Autodesk Inventor part; units mm, degrees
ref_plane "YZ Plane" through (0, 0, 0) normal (1, 0, 0) x (0, 1, 0)
ref_plane "XZ Plane" through (0, 0, 0) normal (0, 1, 0) x (-1, 0, 0)
ref_plane "XY Plane" through (0, 0, 0) normal (0, 0, 1) x (1, 0, 0)
sketch "Sketch1" plane through (0, 0, 0) normal (0, 1, 0) x (-1, 0, 0)
  line L0 (3.5, 3.5) -> (-2.5, 3.5)
  line L1 (-2.5, 3.5) -> (-2.5, -3.5)
  line L2 (-2.5, -3.5) -> (3.5, -3.5)
  line L3 (4.5, -3.5) -> (4.5, 3.5)
  line L4 (4.5, 3.5) -> (4.5, 6.5)
  line L5 (4.5, 6.5) -> (1.5, 6.5)
  line L6 (1.5, 6.5) -> (1.5, 5.5)
  line L7 (1.5, 5.5) -> (3.5, 5.5)
  line L8 (3.5, 5.5) -> (3.5, 3.5)
  line L9 (4.5, -3.5) -> (4.5, -6.5)
  line L10 (4.5, -6.5) -> (1.5, -6.5)
  line L11 (1.5, -6.5) -> (1.5, -5.5)
  line L12 (1.5, -5.5) -> (3.5, -5.5)
  line L13 (3.5, -5.5) -> (3.5, -3.5)
  point P0 (0, 0)
  dimension "d2" = 3.5
  dimension "d3" = 4.5
  dimension "d4" = 1
  dimension "d5" = 1
  dimension "d6" = 2
  dimension "d7" = 2
  dimension "d8" = 7
  dimension "d9" = 7
  dimension "d10" = 1
  dimension "d11" = 1
  dimension "d12" = 3
  dimension "d13" = 3
extrude "Extrusion1" add sketch "Sketch1" along normal blind 120
sketch "Sketch2" plane through (-4.5, 0, -6.5) normal (-1, 0, 0) x (0, 0, 1)
  line L0 (0, 0) -> (13, 0)
  line L1 (0, 0) -> (0, 120)
  point P0 (6.5, 0)
  point P1 (6.5, 60)
  dimension "d16" = 60
  dimension "d17" = 6.5
hole "Hole1" at (-4.5, 60, 0) direction (1, 0, 0) diameter 3.5 end through all
properties part number "Stringer cap"
Input: part model. Units: mm. Frame: model coordinates. A direction names the side the tool comes from. Round coordinates to 2 decimals unless told otherwise and drop trailing zeros. Write each loop counter-clockwise with the first axis right and the second up, starting at its lowest first coordinate (ties: lowest second). Pieces come first, ordered by that corner, then holes.
1) Draft query along Z for faces 1 (the flat face through (-3, 59, 6.5)), 2 (the flat face through (-3, 59, -6.5)), 3 (the flat face through (-2, 0, 0)), 4 (the flat face through (0, 59, -3.5)). Return one class per face: pulls with the +Z half, pulls with the -Z half, needs draft (parallel to the pull), parting line crosses it, or undercut.
2) Contact query for flat-ended pins moving along their axis: P1, Ø0.8, axis at y = 58.5, z = 6, coming from the +X side; P2, Ø1.6, axis at y = 78.5, z = 4.5, coming from the +X side; P3, Ø1, axis at x = 0, y = 60, coming from the +Z side. Output: stop coordinate, or through.
3) Reachability of faces 5 (the flat face through (-2, 120, 0)), 6 (the flat face through (-2, 59, 5.5)) from +Z, -Z, +X, -X, +Y, -Y: full face, straight path, thin tool, end or side. Return the list, or none.
4) Ray query, L1, parallel to Z at x = -2.25, y = 41; L2, parallel to Y at x = -1.25, z = 0; L3, parallel to X at y = 70, z = 5.25. Return the intervals inside material, ascending.
5) Cut plane B-B (z = 0). Return the cut outline in (x, y), then the cut area to 4 significant figures.
6) Cut plane D-D (y = 90). Return the cut outline in (x, z).
7) Cut plane C-C (x = -0.5). Return the cut outline in (y, z), then the cut area to 3 significant figures.
8) Cut plane A-A (y = 60). Return the cut outline in (x, z), then the cut area to 3 significant figures.
Geometry says:
1. face 1: pulls with the +Z half
1. face 2: pulls with the -Z half
1. face 3: needs draft
1. face 4: undercut
2. P1: stops at x = -1.5
2. P2: stops at x = -3.5
2. P3: stops at z = 3.5
3. face 5: +Z, -Z, +X, -X, +Y
3. face 6: +X, +Y, -Y
4. L1: z = -6.5 to -5.5, -3.5 to 3.5, 5.5 to 6.5
4. L2: y = 0 to 58.25, 61.75 to 120
4. L3: x = -4.5 to -3.5
5. outline: (-4.5, 0) - (2.5, 0) - (2.5, 58.25) - (-4.5, 58.25) - close; (-4.5, 61.75) - (2.5, 61.75) - (2.5, 120) - (-4.5, 120) - close
5. area: 815.5 mm2
6. outline: (-4.5, -6.5) - (-1.5, -6.5) - (-1.5, -5.5) - (-3.5, -5.5) - (-3.5, -3.5) - (2.5, -3.5) - (2.5, 3.5) - (-3.5, 3.5) - (-3.5, 5.5) - (-1.5, 5.5) - (-1.5, 6.5) - (-4.5, 6.5) - close
7. outline: (0, -3.5) - (120, -3.5) - (120, 3.5) - (0, 3.5) - close; hole circle Ø3.5 at (60, 0)
7. area: 830 mm2
8. outline: (-4.5, -6.5) - (-1.5, -6.5) - (-1.5, -5.5) - (-3.5, -5.5) - (-3.5, -3.5) - (2.5, -3.5) - (2.5, -1.75) - (-4.5, -1.75) - close; (-4.5, 1.75) - (2.5, 1.75) - (2.5, 3.5) - (-3.5, 3.5) - (-3.5, 5.5) - (-1.5, 5.5) - (-1.5, 6.5) - (-4.5, 6.5) - close
8. area: 34.5 mm2
